Here's how the part is built. I have some questions about the finished solid (model axes, mm). A direction names the side the tool comes from. Round coordinates to 2 decimals unless told otherwise and drop trailing zeros. Write each loop counter-clockwise with the first axis right and the second up, starting at its lowest first coordinate (ties: lowest second). Pieces come first, ordered by that corner, then holes. Notation, with made-up numbers: (30, 9.5) - (76, 9.5) arc R13 ccw to (76, 17.5) - close; hole circle Ø9 at (85, 53). An arc over 180 degrees is marked (long way). One line per item, written item: value. Start each with the question number.
Item 1: For P1, Ø3.5, axis at x = 1.5, z = 4, coming from the +Y side; P2, Ø2, axis at x = 0, z = 0, coming from the -Y side; P3, Ø2, axis at y = 2.5, z = 3.5, coming from the -X side; P4, Ø1, axis at x = 4, y = 7.5, coming from the +Z side, each with a flat end and sliding along its axis, tell me the tip position at first contact or that it passes through.
Item 2: Imagine slicing it at C-C, the plane y = 0.75. Please give me the cut outline in (x, z).
Item 3: If I drill on line 1 (X direction, y = 0.3, z = 0); line 2 (Y direction, x = 2.5, z = 0.5); line 3 (Y direction, x = 5.5, z = -3), over which ranges is the centre line in solid material (lowest first)?
Item 4: For faces 1 (the face through (-3.315, 2.972, 1.879)), 2 (the face through (0, 6, 3)), 3 (the face through (-3, 7, -2)), which set-ups out of +Z, -Z, +X, -X, +Y, -Y let a thin tool reach every point of the face, with its end or its side?
Item 5: Thinking about a two-plate mould opening in X: for faces 4 (the face through (-5.14, 2.96, -4.1)), 5 (the face through (-1.308, 0.507, -1.706)), 6 (the face through (3, 7, -2)), 7 (the face through (-2.1, 6.52, -0.47)), which applies, released by +X, released by -X, zero draft, split by the parting line, or undercut?
Item 6: Imagine slicing it at A-A, the plane y = 7.25. Please give me the cut outline in (x, z).
Item 7: Imagine slicing it at B-B, the plane x = 0. Please give me the cut outline in (y, z).
Item 8: Imagine slicing it at D-D, the plane z = -0.25. Please give me the cut outline in (x, y), then the cut area to 3 significant figures.
```python
from build123d import *

# Parameters (mm, degrees)
SKETCH1_W               = 12
SKETCH1_H               = 10
BOSS_EXTRUDE1_DEPTH     = 1
BOSS_EXTRUDE2_DEPTH     = 4
SKETCH3_W               = 12
SKETCH3_H               = 10
BOSS_EXTRUDE3_DEPTH     = 1
SKETCH5_W               = 12
SKETCH5_H               = 4
BOSS_EXTRUDE4_DEPTH     = 2
SKETCH4_R               = 2.15
CUT_EXTRUDE1_DEPTH      = 10.848857802
CUT_EXTRUDE1_DEPTH_BACK = 10.848857802
FILLET1_R               = 3


with BuildPart() as part:
    # Sketch1 → Boss-Extrude1 (new body)
    with BuildSketch(Plane(origin=(0, 0, 0), x_dir=(1, 0, 0), z_dir=(0, 1, 0))):
        Rectangle(SKETCH1_W, SKETCH1_H)
    extrude(amount=BOSS_EXTRUDE1_DEPTH)

    # Sketch2 → Boss-Extrude2 (add)
    with BuildSketch(Plane(origin=(0, 1, 0), x_dir=(1, 0, 0), z_dir=(0, 1, 0))):
        Polygon((2.2, -3.810511777), (6, -3.810511777), (6, -5), (-6, -5), (-6, 5), (6, 5), (6, 3.810511777), (2.2, 3.810511777), (-2.2, 3.810511777), (-4.4, 0), (-2.2, -3.810511777), align=None)
    extrude(amount=BOSS_EXTRUDE2_DEPTH)

    # Sketch3 → Boss-Extrude3 (add)
    with BuildSketch(Plane(origin=(0, 5, 0), x_dir=(1, 0, 0), z_dir=(0, 1, 0))):
        Rectangle(SKETCH3_W, SKETCH3_H)
    extrude(amount=BOSS_EXTRUDE3_DEPTH)

    # Sketch5 → Boss-Extrude4 (add)
    with BuildSketch(Plane(origin=(0, 6, 0), x_dir=(1, 0, 0), z_dir=(0, 1, 0))):
        Rectangle(SKETCH5_W, SKETCH5_H)
    extrude(amount=BOSS_EXTRUDE4_DEPTH)

    # Sketch4 → Cut-Extrude1 (cut, two sides)
    with BuildSketch(Plane(origin=(0, 6, 0), x_dir=(1, 0, 0), z_dir=(0, 1, 0))) as cut_extrude1_sk:
        with Locations(Location((0, 0, 0), (0, 0, 270))):
            Circle(SKETCH4_R)
    extrude(amount=CUT_EXTRUDE1_DEPTH, mode=Mode.SUBTRACT)
    extrude(cut_extrude1_sk.sketch, amount=-CUT_EXTRUDE1_DEPTH_BACK, mode=Mode.SUBTRACT)

    # Fillet1
    fillet1_edges = [part.edges().sort_by_distance(p)[0] for p in [
        (-6, 3, 5),
        (-6, 3, -5),
    ]]
    fillet(fillet1_edges, radius=FILLET1_R)


solid = part.part
```
Values follow:
1. P1: stops at y = 6
1. P2: passes through
1. P3: stops at x = -5.96
1. P4: stops at z = 2
2. outline: (-6, -2) arc R3 ccw to (-3, -5) - (6, -5) - (6, 5) - (-3, 5) arc R3 ccw to (-6, 2) - close; hole circle Ø4.3 at (0, 0)
3. line 1: x = -6 to -2.15, 2.15 to 6
3. line 2: y = 0 to 1, 5 to 8
3. line 3: y = 0 to 1, 5 to 6
4. face 1: +X
4. face 2: +Z, +X, -X, +Y
4. face 3: -Z, +X, -X, +Y
5. face 4: released by -X
5. face 5: undercut
5. face 6: zero draft
5. face 7: undercut
6. outline: (-6, -2) - (-0.79, -2) arc R2.15 cw to (-0.79, 2) - (-6, 2) - close; (0.79, -2) - (6, -2) - (6, 2) - (0.79, 2) arc R2.15 cw to start
7. outline: (0, -5) - (6, -5) - (6, -2.15) - (5, -2.15) - (5, -3.81) - (1, -3.81) - (1, -2.15) - (0, -2.15) - close; (0, 2.15) - (1, 2.15) - (1, 3.81) - (5, 3.81) - (5, 2.15) - (6, 2.15) - (6, 5) - (0, 5) - close
8. outline: (-6, 0) - (-2.14, 0) - (-2.14, 1) - (-4.26, 1) - (-4.26, 5) - (-2.14, 5) - (-2.14, 8) - (-6, 8) - close; (2.14, 0) - (6, 0) - (6, 1) - (2.14, 1) - close; (2.14, 5) - (6, 5) - (6, 8) - (2.14, 8) - close
8. area: 37.9 mm^2
